```python
from build123d import *

# Parameters (mm, degrees)
F0_W     = 4
F0_H     = 6
F1_DEPTH = 15
F0_W_2   = 2
F2_DEPTH = 24
F0_W_3   = 5
F3_DEPTH = 10
F4_R     = 2.99999
F5_R     = 2.7
F5_R_2   = 0.75
F6_DEPTH = 13.001
F7_D     = 1.1
F7_DEPTH = 40
F7_TIP   = 0.3304733405
F8_R     = 1
F9_DEPTH = 21.001
F10_SIZE = 0.3


# Not quite as in the source:
# - a fillet or chamfer is up to 0.001 mm smaller than in the source, because OpenCascade refuses the exact size


with BuildPart() as f1:
    # F0 (on Front) → F1 (new body)
    with BuildSketch(Plane.XZ):
        with Locations((-9, 39.5)):
            Rectangle(F0_W, F0_H)
    extrude(amount=F1_DEPTH)

    # F0 (on Front) → F2 (join)
    with BuildSketch(Plane.XZ):
        with Locations((-12, 39.5)):
            Rectangle(F0_W_2, F0_H)
        with Locations((-6, 39.5)):
            Rectangle(F0_W_2, F0_H)
    extrude(amount=F2_DEPTH)

    # F0 (on Front) → F3 (join)
    with BuildSketch(Plane.XZ):
        with Locations((-2.5, 39.5)):
            Rectangle(F0_W_3, F0_H)
        Polygon((0, 36.5), (-5, 36.5), (-5, 21), (-10, 21), (-10, 18), (-5, 18), (-5, 0), (0, 0), align=None)
    extrude(amount=F3_DEPTH)

    # F4 (radius 3 in the source; OpenCascade refuses exactly that, so slightly less here)
    f4_edges = [f1.edges().sort_by_distance(p)[0] for p in [
        (-6, -24, 42.5),
        (-6, -24, 36.5),
        (-12, -24, 42.5),
        (-12, -24, 36.5),
    ]]
    fillet(f4_edges, radius=F4_R)

    # F5 (on face) → F6 (cut, through all)
    with BuildSketch(Plane(origin=(-13, 0, 0), x_dir=(0, -1, 0), z_dir=(-1, 0, 0))):
        with Locations((5, 33)):
            Circle(F5_R)
        with Locations((5, 5)):
            Circle(F5_R)
        with Locations((21, 39.5)):
            Circle(F5_R_2)
    extrude(amount=-F6_DEPTH, mode=Mode.SUBTRACT)

    # F7
    with Locations(Plane(origin=(0, 0, 0), x_dir=(1, 0, 0), z_dir=(0, 1, 0))):
        with Locations((-2.5, -33), (-2.5, -5)):
            Hole(F7_D / 2, depth=F7_DEPTH)
            with Locations((0, 0, -(F7_DEPTH + F7_TIP / 2))):  # 118° drill point
                Cone(0, F7_D / 2, F7_TIP, mode=Mode.SUBTRACT)

    # F8 (on face) → F9 (cut, through all)
    with BuildSketch(Plane.XY.offset(21)):
        with Locations((-7.5, -7.5)):
            Circle(F8_R)
    extrude(amount=-F9_DEPTH, mode=Mode.SUBTRACT)

    # F10
    f10_edges = [f1.edges().sort_by_distance(p)[0] for p in [
        (0, -5, 0),
        (0, 0, 21.25),
        (0, -10, 21.25),
        (0, -5, 42.5),
        (0, -2.3, 5),
        (0, -2.3, 33),
    ]]
    chamfer(f10_edges, length=F10_SIZE)


solid = f1.part
```
CAD build for the part. Positions are in the model's coordinates, mm. A direction names the side the tool comes from. Round coordinates to 2 decimals unless told otherwise and drop trailing zeros. Order: outer loops, then holes, each group sorted by start corner. A loop starts at its lowest first (then second) coordinate and runs counter-clockwise, first axis right, second up. Notation, with made-up numbers: (49.25, -10) -> (103.25, -10) arc R21 ccw to (103.25, 10) -> close; hole circle Ø2 at (-24, 1.5). An arc over 180 degrees is marked (long way). One line per question, with ' | ' between items.
Q1. Probe probe 1 along Z at (x, y) = (-1.55, -5); probe 2 along Y at (x, z) = (-1.4, 5); probe 3 along X at (y, z) = (-22.5, 40.5). List the from-to ranges inside material, lowest first.
Completed:
probe 1: z = 0 to 2.3, 7.7 to 30.3, 35.7 to 42.5 | probe 2: y = -10 to -7.7, -2.3 to 0 | probe 3: x = -13 to -11, -7 to -5
Q2. Two-plate mould, pull along Y, no slides. Class faces 1 (the cylindrical face through (-5.99, -23.1, 37.36)), 2 (the cylindrical face through (-2.683, -7.494, 3.966)), 3 (the flat face through (-7, -8, 42.5)): released by +Y, released by -Y, zero draft, split by the parting line, or undercut.
Completed:
face 1: released by -Y | face 2: undercut | face 3: zero draft
Q3. Drop flat-ended pins along their axis: pin 1 (12 mm diameter, centred on y = -12, z = 33, fed in from +X); pin 2 (1.5 mm diameter, centred on x = -2.5, z = 19.5, fed in from -Y); pin 3 (2.5 mm diameter, centred on x = -7.5, y = -7.5, fed in from -Z); pin 4 (5 mm diameter, centred on x = -4.5, y = -15.5, fed in from -Z). Give the stop position or say it passes through.
Completed:
pin 1: stops at x = 0 | pin 2: stops at y = -10 | pin 3: stops at z = 18 | pin 4: stops at z = 36.5
Q4. Which spindle directions (+Z, -Z, +X, -X, +Y, -Y) get a long thin tool onto all of the face, cutting with end or side? Do faces 4 (the cylindrical face through (-2.095, -1.195, 32.628)), 5 (the flat face through (0, -5, 21)), 6 (the flat face through (-9, -8, 36.5)), 7 (the cylindrical face through (-7.63, -6.51, 19.52)), 8 (the flat face through (-10, -5, 20)). Say none if no direction does.
Completed:
face 4: +Y, -Y | face 5: +Z, -Z, +X, +Y, -Y | face 6: -X, +Y, -Y | face 7: -Z | face 8: -Z, -X, +Y, -Y
Q5. Slice it at C-C (x = -7.5). Write the cut outline in (y, z), then the cut area to 3 significant figures.
Completed:
outline: (-15, 36.5) -> (0, 36.5) -> (0, 42.5) -> (-15, 42.5) -> close; (-10, 18) -> (-8.5, 18) -> (-8.5, 21) -> (-10, 21) -> close; (-6.5, 18) -> (0, 18) -> (0, 21) -> (-6.5, 21) -> close | area: 114 mm^2
Q6. Slice it at D-D (y = -15.5). Write the cut outline in (x, z), then the cut area to 3 significant figures.
Completed:
outline: (-13, 36.5) -> (-11, 36.5) -> (-11, 42.5) -> (-13, 42.5) -> close; (-7, 36.5) -> (-5, 36.5) -> (-5, 42.5) -> (-7, 42.5) -> close | area: 24.0 mm^2
Q7. Slice it at A-A (x = -5.5). Give the number of separate pieces and of enclosed holes in the cut face, then the cut area to 3 significant figures.
Completed:
separate pieces: 2 | enclosed holes: 1 | area: 168 mm^2
Q8. Slice it at B-B (y = -5). Write the cut outline in (x, z), then the cut area to 3 significant figures.
Completed:
outline: (-13, 36.5) -> (-5, 36.5) -> (-5, 35.7) -> (-0.3, 35.7) -> (0, 36) -> (0, 42.2) -> (-0.3, 42.5) -> (-13, 42.5) -> close; (-10, 18) -> (-5, 18) -> (-5, 7.7) -> (-0.3, 7.7) -> (0, 8) -> (0, 30) -> (-0.3, 30.3) -> (-5, 30.3) -> (-5, 21) -> (-10, 21) -> close; (-5, 0) -> (-0.3, 0) -> (0, 0.3) -> (0, 2) -> (-0.3, 2.3) -> (-5, 2.3) -> close | area: 221 mm^2
